Can you work these out from the model? Positions are in its coordinate system, mm. A direction names the side the tool comes from. Round coordinates to 2 decimals unless told otherwise and drop trailing zeros. Write each loop counter-clockwise with the first axis right and the second up, starting at its lowest first coordinate (ties: lowest second). Pieces come first, ordered by that corner, then holes. Notation, with made-up numbers: (89.5, 8.5) -> (147.5, 8.5) arc R28 cw to (147.5, 46.5) -> close; hole circle Ø2 at (2, 68.5). An arc over 180 degrees is marked (long way). Write item = value, one per line. Start each with the question number.
1) For faces 4 (the face through (-50.726, 29.353, 64.985)), 5 (the face through (-51, 18, 20)), 6 (the face through (-20.866, -51, 49)), 7 (the face through (19, -36.306, 49)), 8 (the face through (-10, -15, 100)), which set-ups out of +Z, -Z, +X, -X, +Y, -Y let a thin tool reach every point of the face, with its end or its side?
2) Imagine slicing it at B-B, the plane z = 50. Please give me the cut outline in (x, y).
3) Imagine slicing it at C-C, the plane x = -26. Please give me the cut outline in (y, z), then the cut area to 3 significant figures.
4) Imagine slicing it at A-A, the plane y = 9.5. Please give me the cut outline in (x, z).
5) Thinking about a two-plate mould opening in X: for faces 1 (the face through (-40.866, 12, 50)), 2 (the face through (-51, 53.694, 50)), 3 (the face through (59.134, -32, 49)), which applies, +X half, -X half, draft (parallel to the pull), parting line (faces both ways), or undercut?
6) I'm going to push flat-ended pins straight in: pin 1 (20 mm diameter, centred on x = 25, z = 26, fed in from +Y); pin 2 (16 mm diameter, centred on x = -50.5, y = 16, fed in from +Z); pin 3 (22 mm diameter, centred on x = 27.5, y = 22.5, fed in from -Z); pin 4 (10 mm diameter, centred on y = 37.5, z = 50, fed in from -X). Where does each tip first touch, or does it pass through?
7) Imagine slicing it at D-D, the plane x = 35.5. Please give me the cut outline in (y, z), then the cut area to 3 significant figures.
8) If I drill on line 1 (Y direction, x = -56.75, z = 50); line 2 (X direction, y = 47, z = 45); line 3 (Y direction, x = 31.5, z = 11), over which ranges is the centre line in solid material (lowest first)?
from build123d import *

# Parameters (mm, degrees)
BOSS_EXTRUDE1_DEPTH = 100
SKETCH3_W           = 20
SKETCH3_H           = 60
BOSS_EXTRUDE2_DEPTH = 50
FILLET1_R           = 20
SKETCH4_R           = 15
CUT_EXTRUDE1_DEPTH  = 100


with BuildPart() as part:
    # Sketch2 → Boss-Extrude1 (new body)
    with BuildSketch(Plane.XY):
        Polygon((-80.866204042, 3.693693694), (59.133795958, 3.693693694), (59.133795958, -13.693693694), (59.133795958, -66.306306306), (38.267591916, -66.306306306), (-0.866204042, -66.306306306), (-0.866204042, -36.306306306), (39.133795958, -36.306306306), (39.133795958, -16.306306306), (-60.866204042, -16.306306306), (-60.866204042, -36.306306306), (-20.866204042, -36.306306306), (-20.866204042, -66.306306306), (-60, -66.306306306), (-80.866204042, -66.306306306), (-80.866204042, -13.693693694), align=None)
    extrude(amount=BOSS_EXTRUDE1_DEPTH)

    # Sketch3 → Boss-Extrude2 (add)
    with BuildSketch(Plane(origin=(0, 3.693693694, 0), x_dir=(1, 0, 0), z_dir=(0, 1, 0))):
        with Locations((-50.866204042, -50)):
            Rectangle(SKETCH3_W, SKETCH3_H)
        with Locations((29.133795958, -50)):
            Rectangle(SKETCH3_W, SKETCH3_H)
    extrude(amount=BOSS_EXTRUDE2_DEPTH)

    # Fillet1
    fillet1_edges = [part.edges().sort_by_distance(p)[0] for p in [
        (-50.866204042, 53.693693694, 20),
        (-50.866204042, 53.693693694, 80),
        (29.133795958, 53.693693694, 20),
        (29.133795958, 53.693693694, 80),
    ]]
    fillet(fillet1_edges, radius=FILLET1_R)

    # Sketch4 → Cut-Extrude1 (cut)
    with BuildSketch(Plane(origin=(39.133795958, 0, 0), x_dir=(0, 0, -1), z_dir=(1, 0, 0))):
        with Locations((-50, 28.693693694)):
            Circle(SKETCH4_R)
    extrude(amount=-CUT_EXTRUDE1_DEPTH, mode=Mode.SUBTRACT)


solid = part.part
Reported:
q1.face_4 = +X, -X
q1.face_5 = -Z, +X, -X, +Y
q1.face_6 = +Z, -Z, -Y
q1.face_7 = +Z, -Z
q1.face_8 = +Z, +X, -X, +Y, -Y
q2.outline = (-80.87, -66.31) -> (-20.87, -66.31) -> (-20.87, -36.31) -> (-60.87, -36.31) -> (-60.87, -16.31) -> (39.13, -16.31) -> (39.13, -36.31) -> (-0.87, -36.31) -> (-0.87, -66.31) -> (59.13, -66.31) -> (59.13, 3.69) -> (39.13, 3.69) -> (39.13, 13.69) -> (19.13, 13.69) -> (19.13, 3.69) -> (-40.87, 3.69) -> (-40.87, 13.69) -> (-60.87, 13.69) -> (-60.87, 3.69) -> (-80.87, 3.69) -> close; (-60.87, 43.69) -> (-40.87, 43.69) -> (-40.87, 53.69) -> (-60.87, 53.69) -> close; (19.13, 43.69) -> (39.13, 43.69) -> (39.13, 53.69) -> (19.13, 53.69) -> close
q3.outline = (-66.31, 0) -> (-36.31, 0) -> (-36.31, 100) -> (-66.31, 100) -> close; (-16.31, 0) -> (3.69, 0) -> (3.69, 100) -> (-16.31, 100) -> close
q3.area = 5,000 mm²
q4.outline = (-60.87, 20) -> (-40.87, 20) -> (-40.87, 80) -> (-60.87, 80) -> close; (19.13, 20) -> (39.13, 20) -> (39.13, 80) -> (19.13, 80) -> close
q5.face_1 = undercut
q5.face_2 = draft
q5.face_3 = +X half
q6.pin_1 = 53.29
q6.pin_2 = 80
q6.pin_3 = 20
q6.pin_4 = through
q7.outline = (-66.31, 0) -> (-36.31, 0) -> (-36.31, 100) -> (-66.31, 100) -> close; (-16.31, 0) -> (3.69, 0) -> (3.69, 20) -> (33.69, 20) arc R20 ccw to (53.69, 40) -> (53.69, 60) arc R20 ccw to (33.69, 80) -> (3.69, 80) -> (3.69, 100) -> (-16.31, 100) -> close; hole circle Ø30 at (28.69, 50)
q7.area = 7,120 mm²
q8.line_1 = -66.31 to -36.31, -16.31 to 13.69, 43.69 to 53.69
q8.line_2 = -60.87 to -40.87, 19.13 to 39.13
q8.line_3 = -66.31 to -36.31, -16.31 to 3.69
